For this review, take the finished solid that the model builds, in its own axes (mm). Face numbers are marked on the shaded views. A direction names the side the tool comes from. Coordinates: 2 decimals unless noted, no trailing zeros. Write each loop counter-clockwise with the first axis right and the second up, starting at its lowest first coordinate (ties: lowest second). Pieces come first, ordered by that corner, then holes. Notation, with made-up numbers: M -31.75,-38.75 L 5.25,-38.75 A24 ccw 5.25,-21.75 Z; hole C 30.25,-3 d1. An arc over 180 degrees is marked long. Return JSON: item names as keys, results as strings.
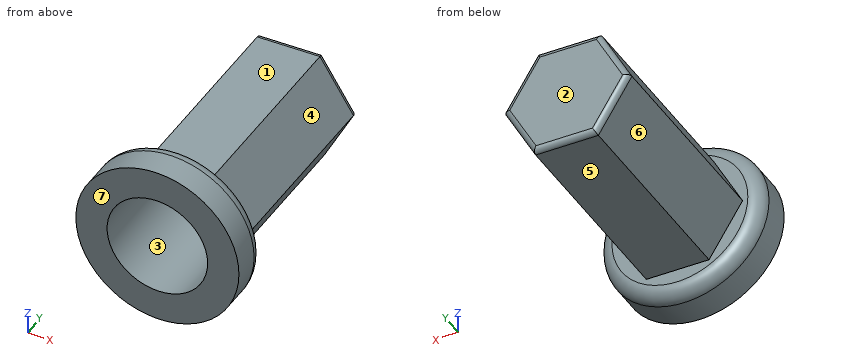
```python
from build123d import *

# Parameters (mm, degrees)
SKETCH1_R           = 7.62
BOSS_EXTRUDE1_DEPTH = 3.81
BOSS_EXTRUDE2_DEPTH = 19.05
FILLET1_R           = 1.27
FILLET2_R           = 0.508
SKETCH3_R           = 4.699
CUT_EXTRUDE1_DEPTH  = 19.05


with BuildPart() as part:
    # Sketch1 → Boss-Extrude1 (new body)
    with BuildSketch(Plane(origin=(0, 0, 0), x_dir=(1, 0, 0), z_dir=(0, 1, 0))):
        Circle(SKETCH1_R)
    extrude(amount=BOSS_EXTRUDE1_DEPTH)

    # Sketch2 → Boss-Extrude2 (add)
    with BuildSketch(Plane(origin=(0, 3.81, 0), x_dir=(1, 0, 0), z_dir=(0, 1, 0))):
        Polygon((5.861093772, -0.236882109), (3.13569281, 4.957415046), (-2.725400962, 5.194297155), (-5.861093772, 0.236882109), (-3.13569281, -4.957415046), (2.725400962, -5.194297155), align=None)
    extrude(amount=BOSS_EXTRUDE2_DEPTH)

    # Fillet1
    fillet1_edges = [part.edges().sort_by_distance(p)[0] for p in [
        (-7.62, 3.81, 0),
    ]]
    fillet(fillet1_edges, radius=FILLET1_R)

    # Fillet2
    fillet2_edges = [part.edges().sort_by_distance(p)[0] for p in [
        (4.293247367, 22.86, 2.715589632),
        (4.498393291, 22.86, -2.360266469),
        (0.205145924, 22.86, -5.0758561),
        (-4.293247367, 22.86, -2.715589632),
        (-4.498393291, 22.86, 2.360266469),
        (-0.205145924, 22.86, 5.0758561),
    ]]
    fillet(fillet2_edges, radius=FILLET2_R)

    # Sketch3 → Cut-Extrude1 (cut)
    with BuildSketch(Plane.XZ):
        Circle(SKETCH3_R)
    extrude(amount=-CUT_EXTRUDE1_DEPTH, mode=Mode.SUBTRACT)


solid = part.part
```
1. Draft analysis for pull direction X (two halves, no side actions). For the marked faces 1, 2 and 3, state which applies: +X half, -X half, draft (parallel to the pull), parting line (faces both ways), or undercut.
Checks:
{"face 1": "-X half", "face 2": "draft", "face 3": "undercut"}
2. For the marked faces 4, 5, 6 and 7, list the 3-axis set-ups (+Z, -Z, +X, -X, +Y, -Y) from which the entire face can be reached by the end or side of a thin tool; tool diameter is ignored.
Checks:
{"face 4": "+Z, +X, +Y", "face 5": "-Z, +X, +Y", "face 6": "-Z, -X, +Y", "face 7": "+Z, -Z, +X, -X, -Y"}
3. Clearance check with flat-ended pins moving along their axes: pin 1 Ø8 at (y, z) = (11, 4.5) entering from +X; pin 2 Ø8 at (x, y) = (-4.5, 4.5) entering from +Z; pin 3 Ø6 at (y, z) = (8, -1) entering from -X. State where each tip first meets the part, or that it passes through.
Checks:
{"pin 1": "x = 5.69", "pin 2": "z = 7.56", "pin 3": "x = -5.86"}
4. Wall thickness on L1, parallel to Y at x = 4.25, z = -3; L2, parallel to X at y = 6, z = 2.25; L3, parallel to Y at x = 0, z = 4: over which ranges is each line inside the solid? List them lowest first. Write a range as from..to.
Checks:
{"L1": "0..3.81", "L2": "-4.56..-4.13, 4.13..4.59", "L3": "19.05..22.86"}
5. We need section A-A (y = 5). State the section outline as (x, z) points.
Checks:
{"outline": "M -5.86,-0.24 L -2.73,-5.19 L 3.14,-4.96 L 5.86,0.24 L 2.73,5.19 L -3.14,4.96 Z; hole C 0,0 d9.4"}
